Design review of the part built by this model. Coordinates are the model's own, in mm. A direction names the side the tool comes from. Give positions to 0.01 mm unless a question says otherwise; leave off trailing zeros. Loops run counter-clockwise (first coordinate to the right, second up) from the corner with the lowest first, then second, coordinate; pieces in that order, holes last. Notation, with made-up numbers: (69, 25.25) -> (103, 25.25) arc R22 ccw to (103, 48.25) -> close; hole circle Ø4 at (-11, 40). An arc over 180 degrees is marked (long way). Use a Markdown table: item, result. Add a question column.
1. For pin 1 Ø4 at (y, z) = (131, -17.5) entering from +X; pin 2 Ø7.5 at (x, y) = (41.5, 102.5) entering from +Z; pin 3 Ø1 at (x, y) = (-4, 103) entering from +Z, all flat-tipped, find the tip position at first contact; note any pin that passes through.
2. Add section C-C (y = 86). State the section outline as (x, z) points, and give its area (3 significant figures).
3. To check wall thickness, follow line 1 (Z direction, x = 45, y = 63.5); line 2 (X direction, y = 40, z = -20); line 3 (Y direction, x = 31.5, z = -57). State the ranges of each line that lie inside material, in increasing order.
4. Add section A-A (x = 30). State the section outline as (y, z) points, and give its area (3 significant figures).
5. Add section D-D (z = -55). State the section outline as (x, y) points.
6. Add section B-B (z = -13). State the section outline as (x, y) points.
7. Draft analysis for pull direction Z (two halves, no side actions). For faces 5 (the flat face through (50, 99, -52)), 6 (the flat face through (38, 15, -55)), 7 (the flat face through (25, 99, -50)), state which applies: pulls with the +Z half, pulls with the -Z half, needs draft (parallel to the pull), parting line crosses it, or undercut.
8. For faces 1 (the flat face through (25, 101, -55)), 2 (the flat face through (-2, 99, 0)), 3 (the flat face through (0, 99, -25)), 4 (the flat face through (-2.5, 99, -12)), list the 3-axis set-ups (+Z, -Z, +X, -X, +Y, -Y) from which the entire face can be reached by the end or side of a thin tool; tool diameter is ignored.
Autodesk Inventor part; units mm, degrees
ref_plane "YZ Plane" through (0, 0, 0) normal (1, 0, 0) x (0, 1, 0)
ref_plane "XZ Plane" through (0, 0, 0) normal (0, 1, 0) x (-1, 0, 0)
ref_plane "XY Plane" through (0, 0, 0) normal (0, 0, 1) x (1, 0, 0)
sketch "Sketch1" plane through (0, 0, 0) normal (0, 1, 0) x (-1, 0, 0)
  line L0 (0, 0) -> (10, 0)
  line L1 (10, 0) -> (10, -60)
  line L2 (10, -60) -> (0, -60)
  line L3 (0, -60) -> (0, 0)
  line L4 (10, -60) -> (-50, -60)
  line L5 (-50, -60) -> (-50, -50)
  line L6 (-50, -50) -> (10, -50)
  line L7 (10, -50) -> (10, -60)
  point P0 (0, -50)
  point P1 (0, -60)
  dimension "d0" = 10
  dimension "d1" = 60
  dimension "d2" = 60
  dimension "d3" = 10
extrude "Extrusion1" add sketch "Sketch1" along normal blind 200
sketch "Sketch2" plane through (-10, 0, 0) normal (0, 0, 1) x (1, 0, 0)
  line L0 (2.5, 15) -> (7.5, 15)
  line L1 (7.5, 15) -> (7.5, 185)
  line L2 (7.5, 185) -> (2.5, 185)
  line L3 (2.5, 185) -> (2.5, 15)
  point P0 (10, 0)
  dimension "d6" = 5
  dimension "d7" = 170
extrude "Extrusion2" cut sketch "Sketch2" against normal blind 25
sketch "Sketch3" plane through (50, 0, -50) normal (1, 0, 0) x (0, 0, -1)
  line L0 (2.5, 15) -> (7.5, 15)
  line L1 (7.5, 15) -> (7.5, 185)
  line L2 (7.5, 185) -> (2.5, 185)
  line L3 (2.5, 185) -> (2.5, 15)
  point P0 (-50, 0)
  dimension "d10" = 5
  dimension "d11" = 170
extrude "Extrusion3" cut sketch "Sketch3" against normal blind 25
properties part number "TSU_FF_Corner_Wall"
Taken from the geometry:
| question | item | result |
|---|---|---|
| 1 | pin 1 | stops at x = 0 |
| 1 | pin 2 | stops at z = -50 |
| 1 | pin 3 | stops at z = -25 |
| 2 | outline | (-10, -60) -> (50, -60) -> (50, -57.5) -> (25, -57.5) -> (25, -52.5) -> (50, -52.5) -> (50, -50) -> (0, -50) -> (0, 0) -> (-2.5, 0) -> (-2.5, -25) -> (-7.5, -25) -> (-7.5, 0) -> (-10, 0) -> close |
| 2 | area | 850 mm^2 |
| 3 | line 1 | z = -60 to -57.5, -52.5 to -50 |
| 3 | line 2 | x = -10 to -7.5, -2.5 to 0 |
| 3 | line 3 | y = 0 to 15, 185 to 200 |
| 4 | outline | (0, -60) -> (200, -60) -> (200, -50) -> (0, -50) -> close; hole (15, -57.5) -> (185, -57.5) -> (185, -52.5) -> (15, -52.5) -> close |
| 4 | area | 1,150 mm^2 |
| 5 | outline | (-10, 0) -> (50, 0) -> (50, 15) -> (25, 15) -> (25, 185) -> (50, 185) -> (50, 200) -> (-10, 200) -> close |
| 6 | outline | (-10, 0) -> (0, 0) -> (0, 200) -> (-10, 200) -> close; hole (-7.5, 15) -> (-2.5, 15) -> (-2.5, 185) -> (-7.5, 185) -> close |
| 7 | face 5 | needs draft |
| 7 | face 6 | undercut |
| 7 | face 7 | pulls with the +Z half |
| 8 | face 1 | +X |
| 8 | face 2 | +Z, +X, -X, +Y, -Y |
| 8 | face 3 | +Z, +X, +Y, -Y |
| 8 | face 4 | +Z |
